from build123d import *

# Parameters (mm, degrees)
F0_W      = 381
F0_H      = 152.4
F1_DEPTH  = 15.875
F3_DEPTH  = 9.525
F4_DEPTH  = 12.7
F5_R      = 3.175
F6_R      = 4
F7_DEPTH  = 5
F8_W      = 76.2
F8_H      = 9.525
F9_DEPTH  = 6.35
F10_R     = 6.34999
F11_R     = 5
F12_DEPTH = 15
F13_R     = 3.175


# Not quite as in the source:
# - a fillet or chamfer is up to 0.001 mm smaller than in the source, because OpenCascade refuses the exact size
# - ends of sketch curves that miss each other by under 0.0002 mm in the source are joined


with BuildPart() as f1:
    # F0 (on Top) → F1 (new body)
    with BuildSketch(Plane.XY):
        Rectangle(F0_W, F0_H)
    extrude(amount=-F1_DEPTH)

    # F2 (on face) → F3 (cut)
    with BuildSketch(Plane.XY):
        Polygon((-69.85, -25.4), (-69.85, 0), (-69.85, 25.4), (-120.65, 25.4), (-120.65, -25.4), align=None)
    extrude(amount=-F3_DEPTH, mode=Mode.SUBTRACT)

    # F2 (on face) → F4 (cut)
    with BuildSketch(Plane.XY):
        Polygon((47.625, 0), (47.625, -34.925), (142.875, -34.925), (142.875, 34.925), (47.625, 34.925), align=None)
    extrude(amount=-F4_DEPTH, mode=Mode.SUBTRACT)

    # F5
    f5_edges = [f1.edges().sort_by_distance(p)[0] for p in [
        (-69.85, 25.4, -4.7625),
        (142.875, 34.925, -6.35),
        (-69.85, -25.4, -4.7625),
        (142.875, -34.925, -6.35),
        (-120.65, -25.4, -4.7625),
        (47.625, -34.925, -6.35),
        (47.625, 34.925, -6.35),
        (-120.65, 25.4, -4.7625),
    ]]
    fillet(f5_edges, radius=F5_R)

    # F6 (on face) → F7 (cut)
    with BuildSketch(Plane.XY):
        with Locations((-171.4581174665, -57.1581174665)):
            Circle(F6_R)
        with Locations((171.4581174665, -57.1581174665)):
            Circle(F6_R)
    extrude(amount=-F7_DEPTH, mode=Mode.SUBTRACT)

    # F8 (on face) → F9 (cut)
    with BuildSketch(Plane.XZ.offset(76.2)):
        with Locations((0, -4.7625)):
            Rectangle(F8_W, F8_H)
    extrude(amount=-F9_DEPTH, mode=Mode.SUBTRACT)

    # F10 (radius 6.35 in the source; OpenCascade refuses exactly that, so slightly less here)
    f10_edges = [f1.edges().sort_by_distance(p)[0] for p in [
        (-38.1, -73.025, -9.525),
        (-38.1, -69.85, -4.7625),
        (0, -69.85, -9.525),
        (38.1, -73.025, -9.525),
        (38.1, -69.85, -4.7625),
    ]]
    fillet(f10_edges, radius=F10_R)

    # F11 (on face) → F12 (cut)
    with BuildSketch(Plane.XY):
        with Locations((-171.45, 66.675)):
            Circle(F11_R)
        with Locations((171.45, 66.675)):
            Circle(F11_R)
    extrude(amount=-F12_DEPTH, mode=Mode.SUBTRACT)

    # F13
    f13_edges = [f1.edges().sort_by_distance(p)[0] for p in [
        (-190.5, -76.2, -7.9375),
        (190.5, -76.2, -7.9375),
        (190.5, 76.2, -7.9375),
        (-190.5, 76.2, -7.9375),
    ]]
    fillet(f13_edges, radius=F13_R)

    # F14 (on face) → F15 (revolve, cut)
    with BuildSketch(Plane.XY):
        with BuildLine():
            Line((47.625, -12.7), (47.625, 12.7))
            ThreePointArc((47.625, 12.7), (34.925, 1.535e-07), (47.625, -12.7))
        make_face()
    revolve(axis=Axis((47.625, 0, 0), (0, -1, 0)), mode=Mode.SUBTRACT)


solid = f1.part
Source: CAD feature listing. Evaluate the final solid. Frame: model axes, mm. A direction names the side the tool comes from. Round coordinates to 2 decimals unless told otherwise and drop trailing zeros. Write each loop counter-clockwise with the first axis right and the second up, starting at its lowest first coordinate (ties: lowest second). Pieces come first, ordered by that corner, then holes. Notation, with made-up numbers: (45, 44) - (88, 44) arc R27 cw to (88, 72) - close; hole circle Ø6 at (56, 84). An arc over 180 degrees is marked (long way). Use CSV: the item, a comma, the result in double quotes. Start each with the question number.
(1) Cut plane C-C, the plane x = -107. Return loops of the section in (y, z) (3 decimals), and give its area (3 significant figures).
(2) Set-up query: faces 1 (the face through (0.445, -71.661, -7.615)), 2 (the face through (-96, -25.4, -5)), 3 (the face through (-3, 1, 0)). Return all of +Z, -Z, +X, -X, +Y, -Y with unobstructed straight access to the full face (end or side cutting, diameter ignored); none if empty.
(3) Cut plane B-B, the plane x = 107. Return loops of the section in (y, z) (3 decimals), and give its area (3 significant figures).
(4) Mould query, pull axis X, two halves, no side actions, for faces 4 (the face through (-3, 76.2, -8)), 5 (the face through (-190.5, -1, -8)), 6 (the face through (-175.14, 70.05, -7.4)). Classes: pulls with the +X half, pulls with the -X half, needs draft (parallel to the pull), parting line crosses it, or undercut.
(5) Material intervals for probe 1 along X at (y, z) = (-17, -0.75) (3 decimals); probe 2 along X at (y, z) = (66, -10); probe 3 along X at (y, z) = (26, -10) (3 decimals), sorted ascending. Write a range as [from, to].
(6) First-contact query: pin 1 Ø9 at (x, y) = (171.45, 66.675) entering from +Z; pin 2 Ø21 at (x, y) = (103, -0.5) entering from +Z. Flat tips, straight axial feed; report the tip coordinate or a pass-through.
(7) Cut plane A-A, the plane x = 171.45. Return loops of the section in (y, z) (3 decimals).
Geometry says:
1,outline,"(-76.2, -15.875) - (76.2, -15.875) - (76.2, 0) - (25.4, 0) - (25.4, -9.525) - (-25.4, -9.525) - (-25.4, 0) - (-76.2, 0) - close"
1,area,"1,940 mm²"
2,face 1,"+Z, -Y"
2,face 2,"+Z"
2,face 3,"+Z, +X, -X, +Y, -Y"
3,outline,"(-76.2, -15.875) - (76.2, -15.875) - (76.2, 0) - (34.925, 0) - (34.925, -12.7) - (-34.925, -12.7) - (-34.925, 0) - (-76.2, 0) - close"
3,area,"1,530 mm²"
4,face 4,"needs draft"
4,face 5,"pulls with the -X half"
4,face 6,"undercut"
5,probe 1,"[-190.5, -120.65], [-69.85, 47.625], [142.875, 190.5]"
5,probe 2,"[-190.5, -176.4], [-166.5, 166.5], [176.4, 190.5]"
5,probe 3,"[-190.5, 47.625], [142.875, 190.5]"
6,pin 1,"z = -15"
6,pin 2,"z = -12.7"
7,outline,"(-76.2, -15.875) - (76.2, -15.875) - (76.2, 0) - (71.675, 0) - (71.675, -15) - (61.675, -15) - (61.675, 0) - (-53.158, 0) - (-53.158, -5) - (-61.158, -5) - (-61.158, 0) - (-76.2, 0) - close"
